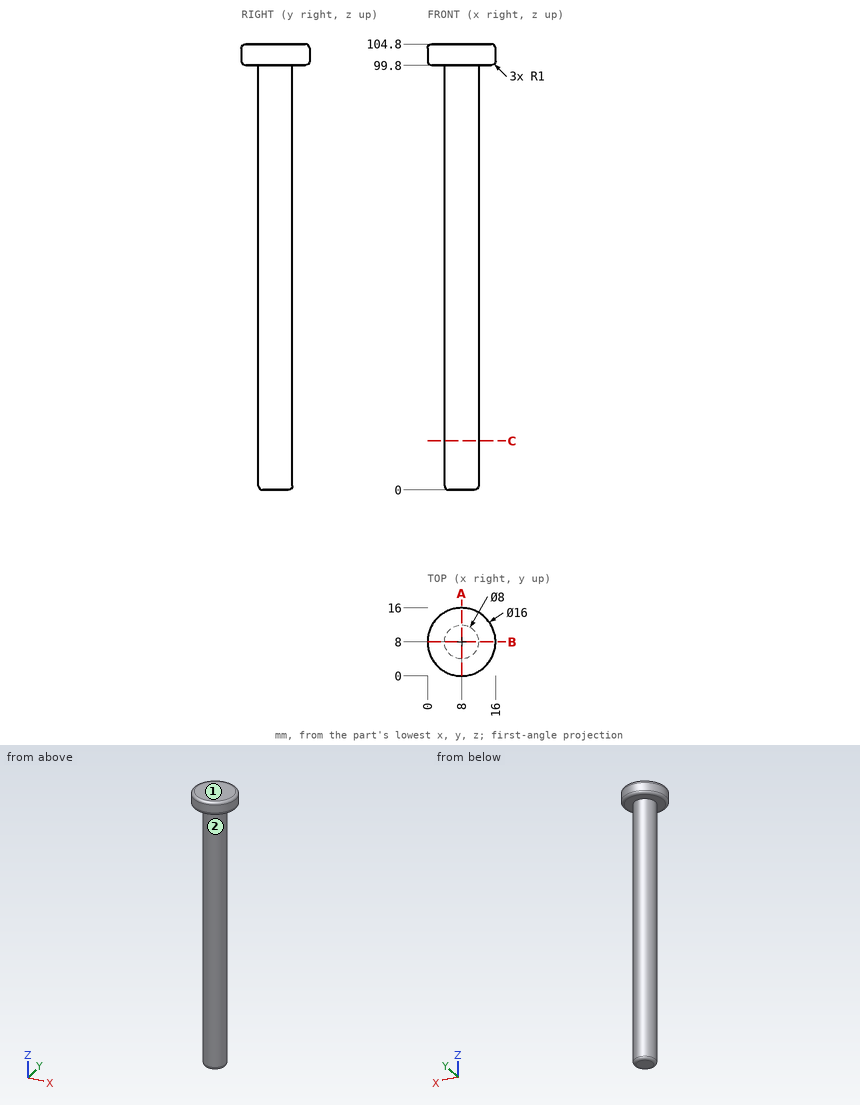
The figure shows three views and two pictorial views of one solid part (mm, origin at its lowest corner). Answer the questions. A direction names the side the tool comes from. Coordinates: 2 decimals unless noted, no trailing zeros. Write each loop counter-clockwise with the first axis right and the second up, starting at its lowest first coordinate (ties: lowest second). Pieces come first, ordered by that corner, then holes.
1. The part is cut by section C-C, the plane z = 11.5. Write down the section's boundary in (x, y), and give its area (3 significant figures).
Results list:
outline: circle Ø8 at (8, 8)
area: 50.3 mm2
2. The part is cut by section A-A, the plane x = 8. Write down the section's boundary in (y, z).
Results list:
outline: (0, 100.8) arc R1 ccw to (1, 99.8) - (4, 99.8) - (4, 1) arc R1 ccw to (5, 0) - (11, 0) arc R1 ccw to (12, 1) - (12, 99.8) - (15, 99.8) arc R1 ccw to (16, 100.8) - (16, 103.8) arc R1 ccw to (15, 104.8) - (1, 104.8) arc R1 ccw to (0, 103.8) - close
3. Consider line 1 along Z through (x, y) = (7.75, 13); line 2 along Z through (x, y) = (14.25, 4); line 3 along Y through (x, z) = (7.75, 58). Determine where each line is inside the solid, lowest interval first.
Results list:
line 1: z = 99.8 to 104.8
line 2: z = 99.89 to 104.71
line 3: y = 4.01 to 11.99
4. Flat-ended cylindrical pins translate along their axes: pin 1 (6 mm diameter, centred on x = 4.5, z = 39.5, fed in from +Y); pin 2 (1 mm diameter, centred on x = 12, y = 6.5, fed in from -Z); pin 3 (4 mm diameter, centred on x = 13.5, z = 90, fed in from -Y). Find the tip coordinate at first contact, or state that the pin passes through.
Results list:
pin 1: stops at y = 11.97
pin 2: stops at z = 0.36
pin 3: stops at y = 6.06
5. For the marked faces 1 and 2, determine the directions among +Z, -Z, +X, -X, +Y, -Y from which every point of the face is accessible in a straight line to the end or side of a thin tool.
Results list:
face 1: +Z, +X, -X, +Y, -Y
face 2: -Z
